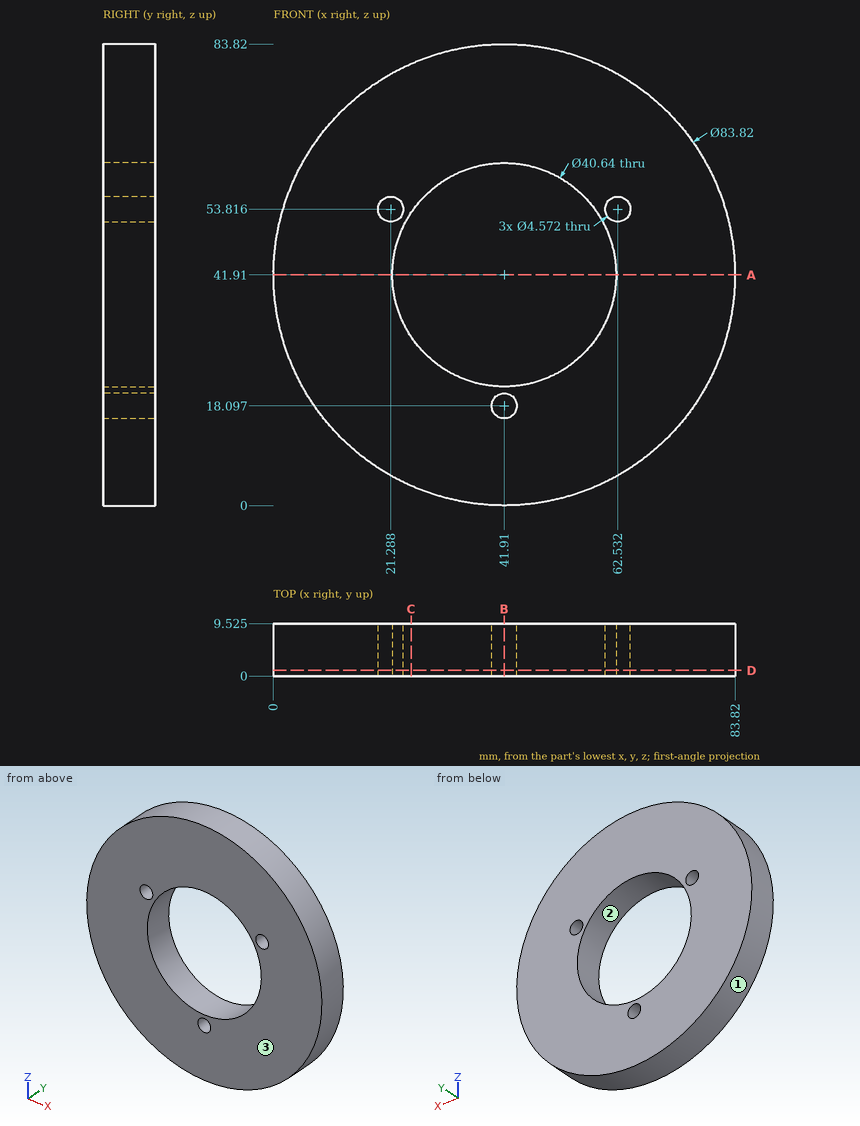
Study the drawing (mm; zero at the part's minimum x, y, z) and answer. Coordinates: 2 decimals unless noted, no trailing zeros. Write each loop counter-clockwise with the first axis right and the second up, starting at its lowest first coordinate (ties: lowest second). Pieces come first, ordered by that corner, then holes. Notation, with made-up numbers: M 34,7.25 L 57,7.25 A30 cw 57,45.25 Z; hole C 8,14.25 d8. An arc over 180 degrees is marked long. Use one line per item in the form item = value.
Item 1: The mould has two halves that part along X. Classify the marked faces 1, 2 and 3: released by +X, released by -X, zero draft, split by the parting line, or undercut.
Model answer:
face_1 = split by the parting line
face_2 = undercut
face_3 = zero draft
Item 2: Find section C-C, the plane x = 25. Give the vertices of the cut face in (y, z) (1 decimal).
Model answer:
outline = M 0,3.6 L 9.5,3.6 L 9.5,30.6 L 0,30.6 Z; M 0,53.2 L 9.5,53.2 L 9.5,80.3 L 0,80.3 Z
Item 3: Find section A-A, the plane z = 41.91. Give the vertices of the cut face in (x, y) (1 decimal).
Model answer:
outline = M 0,0 L 21.6,0 L 21.6,9.5 L 0,9.5 Z; M 62.2,0 L 83.8,0 L 83.8,9.5 L 62.2,9.5 Z
Item 4: Find the intervals of material crossed by probe 1 along X at (y, z) = (6.5, 42); probe 2 along Z at (x, y) = (36, 8.25); probe 3 along Z at (x, y) = (43, 1) (1 decimal), in increasing order.
Model answer:
probe_1 = 0 to 21.59, 62.23 to 83.82
probe_2 = 0.42 to 22.47, 61.35 to 83.4
probe_3 = 0 to 16.1, 20.1 to 21.6, 62.2 to 83.8
Item 5: Find section D-D, the plane y = 1. Give the vertices of the cut face in (x, z) (1 decimal), plus the area to 3 significant figures.
Model answer:
outline = C 41.9,41.9 d83.8; hole C 21.3,53.8 d4.6; hole C 41.9,41.9 d40.6; hole C 41.9,18.1 d4.6; hole C 62.5,53.8 d4.6
area = 4,170 mm2
Item 6: Find section B-B, the plane x = 41.91. Give the vertices of the cut face in (y, z) (1 decimal).
Model answer:
outline = M 0,0 L 9.5,0 L 9.5,15.8 L 0,15.8 Z; M 0,20.4 L 9.5,20.4 L 9.5,21.6 L 0,21.6 Z; M 0,62.2 L 9.5,62.2 L 9.5,83.8 L 0,83.8 Z
Item 7: Given P1, Ø4, axis at y = 1.5, z = 13, coming from the -X side; P2, Ø2.5, axis at x = 62.53, z = 53.82, coming from the -Y side; P3, Ø4, axis at x = 61.5, y = 4.5, coming from the -Z side; P4, Ø10, axis at x = 17.5, z = 11.5, coming from the -Y side, each flat-ended and moving along its own axis, determine where each tip first touches the part or whether it passes through.
Model answer:
P1 = 9.78
P2 = through
P3 = 3.87
P4 = 0
